Input: part model. Units: mm. Frame: model coordinates. A direction names the side the tool comes from. Give positions to 0.01 mm unless a question says otherwise; leave off trailing zeros. Loops run counter-clockwise (first coordinate to the right, second up) from the corner with the lowest first, then second, coordinate; pieces in that order, holes last. Notation, with made-up numbers: (19, 53.5) -> (64, 53.5) arc R25 ccw to (64, 72.5) -> close; hole circle Ø10 at (43, 87). An arc over 180 degrees is marked (long way). Answer in a Markdown table with one row per item. Add a question column.
```python
from build123d import *

# Parameters (mm, degrees)
SKETCH1_R           = 32.5
SKETCH1_R_2         = 25
BOSS_EXTRUDE1_DEPTH = 25
SKETCH2_R           = 10
BOSS_EXTRUDE3_DEPTH = 25
SKETCH4_R           = 2
CUT_EXTRUDE1_DEPTH  = 10
BOSS_EXTRUDE5_DEPTH = 5
FILLET4_R           = 4


with BuildPart() as part:
    # Sketch1 → Boss-Extrude1 (new body)
    with BuildSketch(Plane(origin=(0, 0, 0), x_dir=(1, 0, 0), z_dir=(0, 1, 0))):
        with Locations(Location((0, 0, 0), (0, 0, 270))):
            Circle(SKETCH1_R)
        with Locations(Location((0, 0, 0), (0, 0, 270))):
            Circle(SKETCH1_R_2, mode=Mode.SUBTRACT)
    extrude(amount=BOSS_EXTRUDE1_DEPTH)



with BuildPart() as body_2:
    # Sketch2 → Boss-Extrude3 (new body)
    with BuildSketch(Plane(origin=(0, 25, 0), x_dir=(1, 0, 0), z_dir=(0, 1, 0))):
        with Locations(Location((0, 0, 0), (0, 0, 270))):
            Circle(SKETCH2_R)
    extrude(amount=-BOSS_EXTRUDE3_DEPTH)

    # Sketch4 → Cut-Extrude1 (cut)
    with BuildSketch(Plane(origin=(0, 25, 0), x_dir=(1, 0, 0), z_dir=(0, 1, 0))):
        with Locations(Location((0, 0, 0), (0, 0, 270))):
            Circle(SKETCH4_R)
    extrude(amount=-CUT_EXTRUDE1_DEPTH, mode=Mode.SUBTRACT)


with BuildPart() as part_1:
    add(part.part)

    add(body_2.part)  # Boss-Extrude5 merges body 2
    # Sketch6 → Boss-Extrude5 (add)
    with BuildSketch(Plane(origin=(0, 0, 0), x_dir=(-1, 0, 0), z_dir=(0, -1, 0))):
        with BuildLine():
            Line((3.5, 3.5), (3.5, 25))
            ThreePointArc((3.5, 25), (0, 28.5), (-3.5, 25))
            Line((-3.5, 25), (-3.5, 3.5))
            Line((-3.5, 3.5), (3.5, 3.5))
        make_face()
        with BuildLine():
            Line((25, 3.5), (3.5, 3.5))
            Line((3.5, 3.5), (3.5, -3.5))
            Line((3.5, -3.5), (25, -3.5))
            ThreePointArc((25, -3.5), (28.5, 0), (25, 3.5))
        make_face()
        with BuildLine():
            Line((3.5, -25), (3.5, -3.5))
            Line((3.5, -3.5), (-3.5, -3.5))
            Line((-3.5, -3.5), (-3.5, -25))
            ThreePointArc((-3.5, -25), (0, -28.5), (3.5, -25))
        make_face()
        with BuildLine():
            Line((-3.5, -3.5), (-3.5, 3.5))
            Line((-3.5, 3.5), (-25, 3.5))
            ThreePointArc((-25, 3.5), (-28.5, 0), (-25, -3.5))
            Line((-25, -3.5), (-3.5, -3.5))
        make_face()
    extrude(amount=-BOSS_EXTRUDE5_DEPTH)

    # Fillet4
    fillet4_edges = [part_1.edges().sort_by_distance(p)[0] for p in [
        (0, 0, -32.5),
        (0, 25, -32.5),
    ]]
    fillet(fillet4_edges, radius=FILLET4_R)


solid = part_1.part
```
1) Reachability of faces 1 (the face through (3.5, 2, -17)), 2 (the face through (0, 15, 0)), 3 (the face through (2.4, 25, -0.1)) from +Z, -Z, +X, -X, +Y, -Y: full face, straight path, thin tool, end or side. Return the list, or none.
2) Material intervals for line 1 along X through (y, z) = (15.5, 0); line 2 along X through (y, z) = (10.25, 0), sorted ascending.
3) Pin query (flat end, axial travel): pin 1 (8 mm diameter, centred on x = -23, z = -6, fed in from -Y); pin 2 (2 mm diameter, centred on y = 7.5, z = 14, fed in from -X); pin 3 (5 mm diameter, centred on y = 2.5, z = 11, fed in from +X); pin 4 (4 mm diameter, centred on y = 2, z = 18, fed in from -X). Return the tip coordinate at first contact, or that it passes through.
4) Pull-direction query (X, two-part tool) for faces 4 (the face through (9.76, 12.38, 31)), 5 (the face through (-3.5, 2, -17)), 6 (the face through (0, 0, 0)); classes: +X half, -X half, draft (parallel to the pull), parting line (faces both ways), or undercut.
5) Section B-B on z = 0. Output: boundary loops of the cut face in (x, y), and give its area (3 significant figures).
6) Section C-C on y = 8.75. Output: boundary loops of the cut face in (x, z).
7) Section A-A on y = 19.75. Output: boundary loops of the cut face in (x, z).
8) Section D-D on x = 0. Output: boundary loops of the cut face in (y, z).
Working result:
| question | item | result |
|---|---|---|
| 1 | face 1 | +Y, -Y |
| 1 | face 2 | +Y |
| 1 | face 3 | +Z, -Z, +X, -X, +Y |
| 2 | line 1 | x = -32.5 to -25, -10 to -2, 2 to 10, 25 to 32.5 |
| 2 | line 2 | x = -32.5 to -25, -10 to 10, 25 to 32.5 |
| 3 | pin 1 | stops at y = 0 |
| 3 | pin 2 | stops at x = -29.79 |
| 3 | pin 3 | stops at x = 31.28 |
| 3 | pin 4 | stops at x = -27.99 |
| 4 | face 4 | parting line |
| 4 | face 5 | undercut |
| 4 | face 6 | draft |
| 5 | outline | (-32.5, 4) arc R4 ccw to (-28.5, 0) -> (28.5, 0) arc R4 ccw to (32.5, 4) -> (32.5, 21) arc R4 ccw to (28.5, 25) -> (25, 25) -> (25, 5) -> (10, 5) -> (10, 25) -> (2, 25) -> (2, 15) -> (-2, 15) -> (-2, 25) -> (-10, 25) -> (-10, 5) -> (-25, 5) -> (-25, 25) -> (-28.5, 25) arc R4 ccw to (-32.5, 21) -> close |
| 5 | area | 971 mm2 |
| 6 | outline | circle Ø65 at (0, 0); circle Ø20 at (0, 0); hole circle Ø50 at (0, 0) |
| 7 | outline | circle Ø65 at (0, 0); circle Ø20 at (0, 0); hole circle Ø50 at (0, 0); hole circle Ø4 at (0, 0) |
| 8 | outline | (0, -28.5) arc R4 ccw to (4, -32.5) -> (21, -32.5) arc R4 ccw to (25, -28.5) -> (25, -25) -> (5, -25) -> (5, -10) -> (25, -10) -> (25, -2) -> (15, -2) -> (15, 2) -> (25, 2) -> (25, 10) -> (5, 10) -> (5, 25) -> (25, 25) -> (25, 28.5) arc R4 ccw to (21, 32.5) -> (4, 32.5) arc R4 ccw to (0, 28.5) -> close |
